Model file for the job. Use its own axes, mm. A direction names the side the tool comes from. Round coordinates to 2 decimals unless told otherwise and drop trailing zeros. Order: outer loops, then holes, each group sorted by start corner. A loop starts at its lowest first (then second) coordinate and runs counter-clockwise, first axis right, second up. Notation, with made-up numbers: (33, 57.25) -> (49, 57.25) arc R24 cw to (49, 70.25) -> close; hole circle Ø6 at (60, 89.5). An arc over 180 degrees is marked (long way). Put each result on its own line as item: value. Start each with the question number.
Q1. Cut at B-B, the plane x = 20. List the corners of the cut face in (y, z), and give its area (3 significant figures).
Q2. Cut at D-D, the plane x = 75. List the corners of the cut face in (y, z).
Q3. Pull direction Y, two halves, no side cores. Call faces 4 (the face through (31.45, -6.18, 6.44)), 5 (the face through (40.191, -13.594, 0.376)), 6 (the face through (62.31, -6.26, 7.31)): released by +Y, released by -Y, zero draft, split by the parting line, or undercut.
Q4. 3-axis set-ups, long thin cutter, end or side, ignore diameter. For faces 1 (the face through (13, 0, 6)), 2 (the face through (76, -6, 12.7)), 3 (the face through (69, 0, 6)): which of +Z, -Z, +X, -X, +Y, -Y reach the whole face in a straight line?
Q5. Probe L1, parallel to Z at x = 75, y = -6.5; L2, parallel to X at y = -6, z = 10.75; L3, parallel to X at y = -5, z = 6.35. List the from-to ranges inside material, lowest first.
Q6. Cut at A-A, the plane y = -6.35. State how many separate pieces and enclosed holes the cut face has, and give its area (3 significant figures).
Q7. Flat gauge pins, fed straight in: P1, Ø1, axis at x = 35, y = -11.5, coming from the +Z side; P2, Ø6.5, axis at x = 67.5, z = 7.5, coming from the +Y side; P3, Ø2, axis at y = -2.5, z = 3.5, coming from the -X side; P4, Ø4, axis at x = 60, z = 6.35, coming from the -Y side. Where does each tip first touch, or does it go through?
Q8. Cut at C-C, the plane x = 66. List the corners of the cut face in (y, z).
Autodesk Fusion 360 part; units mm, degrees
sketch "Screw Holes" plane through (0, 0, 0) normal (0, 1, 0) x (1, 0, 0)
  line L0 (0, 0) -> (80, 0)
  line L1 (80, 0) -> (80, -12.7)
  line L2 (80, -12.7) -> (0, -12.7)
  line L3 (0, -12.7) -> (0, 0)
  line L4 (0, -6.35) -> (80, -6.35) construction
  circle A0 centre (5, -6.35) radius 2
  circle A1 centre (20, -6.35) radius 2
  circle A2 centre (60, -6.35) radius 2.5
  circle A3 centre (75, -6.35) radius 2.5
  line L5 (5, -6.35) -> (0, -6.35)
  line L6 (75, -6.35) -> (80, -6.35)
  line L7 (5, -6.35) -> (20, -6.35) construction
  line L8 (60, -6.35) -> (75, -6.35) construction
  point P0 (67.5, -6.35)
  point P1 (12.5, -6.35)
  dimension "d1" = 80
  dimension "d2" = 12.7
  dimension "d3" = 4
  dimension "d4" = 4
  dimension "d5" = 5
  dimension "d6" = 5
  dimension "d7" = 40
  dimension "d8" = 15
  dimension "d9" = 15
extrude "Extrude1" add sketch "Screw Holes" against normal blind 12.7 contours A0 | A3 | L0 L1 L2 L3 | A1 | A2
extrude "Extrude2" cut sketch "Screw Holes" against normal through all contours A0 | A3 | A1 | A2
sketch "Loadcell Holes" plane through (0, 0, 12.7) normal (0, 0, 1) x (1, 0, 0)
  line L0 (80, 0) -> (0, 0)
  line L1 (0, 0) -> (0, -12.7)
  line L2 (0, -12.7) -> (80, -12.7)
  line L3 (80, -12.7) -> (80, 0)
  line L4 (40, -12.7) -> (40, 0) construction
  line L5 (0, -6.35) -> (80, -6.35) construction
  circle A0 centre (36.936, -6.35) radius 5.4886
  circle A1 centre (43.064, -6.35) radius 5.4886
  line L6 (36.936, -6.35) -> (43.064, -6.35)
extrude "Extrude3" cut sketch "Loadcell Holes" against normal blind 25 contours A0 A1 L6 | A0 A1 | A0 A1 L6 | A0 A1
sketch "Arrow" plane through (0, 0, 0) normal (-1, 0, 0) x (0, 0, 1)
  line L0 (12.7, 0) -> (0, 0)
  line L1 (0, 0) -> (0, -12.7)
  line L2 (0, -12.7) -> (12.7, -12.7)
  line L3 (12.7, -12.7) -> (12.7, 0)
  line L4 (5.511, -2.3504) -> (7.189, -2.3504)
  line L5 (7.189, -2.3504) -> (7.189, -8.0971)
  line L6 (7.189, -8.0971) -> (9.0409, -8.0971)
  line L7 (9.0409, -8.0971) -> (6.35, -10.7879)
  line L8 (6.35, -10.7879) -> (3.6591, -8.0971)
  line L9 (3.6591, -8.0971) -> (5.511, -8.0971)
  line L10 (5.511, -8.0971) -> (5.511, -2.3504)
  line L11 (6.35, -12.7) -> (6.35, 0) construction
  dimension "d20" = 45
extrude "Extrude4" cut sketch "Arrow" against normal blind 0.25 contours L4 L5 L6 L7 L8 L9 L10
sketch "Sketch5" plane through (0, 0, 0) normal (0, 1, 0) x (1, 0, 0)
  circle A0 centre (20, -6.35) radius 2
  circle A1 centre (60, -6.35) radius 2.5
  circle A2 centre (5, -6.35) radius 2
  circle A3 centre (75, -6.35) radius 2.5
  line L0 (80, -12.7) -> (80, 0)
  line L1 (80, 0) -> (0, 0)
  line L2 (0, 0) -> (0, -12.7)
  line L3 (0, -12.7) -> (80, -12.7)
  line L4 (40, 0) -> (40, -12.7) construction
  line L5 (26.35, 0) -> (53.65, 0)
  line L6 (53.65, 0) -> (53.65, -12.7)
  line L7 (53.65, -12.7) -> (26.35, -12.7)
  line L8 (26.35, -12.7) -> (26.35, 0)
  line L9 (26.35, -6.35) -> (40, -6.35) construction
  line L10 (40, -6.35) -> (53.65, -6.35) construction
  circle A4 centre (20, -6.35) radius 6.35 construction
extrude "Extrude6" add sketch "Sketch5" along normal blind 1.25 contours L1 L3 L5 L6 L7 L8
fillet "Fillet1" radius 1.25 4 edges at (26.35, 1.25, 6.35) (40, 1.25, 12.7) (53.65, 1.25, 6.35) (40, 1.25, 0)
sketch "Sketch6" plane through (0, -12.7, 0) normal (0, -1, 0) x (1, 0, 0)
  line L0 (80, 0) -> (80, 12.7)
  line L1 (80, 12.7) -> (0, 12.7)
  line L2 (0, 12.7) -> (0, 0)
  line L3 (0, 0) -> (80, 0)
  line L4 (26.35, 12.7) -> (26.35, 0)
  line L5 (26.35, 0) -> (0, 0)
  line L6 (0, 0) -> (0, 12.7)
  line L7 (0, 12.7) -> (26.35, 12.7)
  circle A0 centre (20, 6.35) radius 2
  circle A1 centre (5, 6.35) radius 2
  line L8 (53.65, 0) -> (53.65, 12.7)
  line L9 (53.65, 12.7) -> (80, 12.7)
  line L10 (80, 12.7) -> (80, 0)
  line L11 (80, 0) -> (53.65, 0)
  circle A2 centre (75, 6.35) radius 2.5
  circle A3 centre (60, 6.35) radius 2.5
  circle A4 centre (20, 6.35) radius 2
  circle A5 centre (60, 6.35) radius 2.5
  circle A6 centre (5, 6.35) radius 2
  circle A7 centre (75, 6.35) radius 2.5
  line L12 (5, 6.35) -> (20, 6.35) construction
  line L13 (60, 6.35) -> (75, 6.35) construction
  point P0 (67.5, 6.35)
  point P1 (12.5, 6.35)
extrude "Extrude7" add sketch "Sketch6" along normal blind 1.25 contours L1 L3 L4 L8
fillet "Fillet2" radius 1.25 4 edges at (26.35, -13.95, 6.35) (40, -13.95, 0) (53.65, -13.95, 6.35) (40, -13.95, 12.7)
sketch "Sketch7" plane through (0, 0, 12.7) normal (0, 0, 1) x (1, 0, 0)
  line L0 (26.35, -12.7) -> (53.65, -12.7)
  line L1 (53.65, -12.7) -> (80, -12.7)
  line L2 (80, -12.7) -> (80, 0)
  line L3 (80, 0) -> (53.65, 0)
  line L4 (53.65, 0) -> (26.35, 0)
  line L5 (26.35, 0) -> (0, 0)
  line L6 (0, 0) -> (0, -12.7)
  line L7 (0, -12.7) -> (26.35, -12.7)
  arc A0 (40, -1.7962) -> (40, -10.9038) centre (36.936, -6.35) ccw
  arc A1 (40, -10.9038) -> (40, -1.7962) centre (43.064, -6.35) ccw
  line L8 (51, 0) -> (72.1962, 0)
  line L9 (72.1962, 0) -> (72.1962, -12.7)
  line L10 (72.1962, -12.7) -> (51, -12.7)
  line L11 (51, -12.7) -> (51, 0)
extrude "Extrude8" add sketch "Sketch7" along normal blind 1.25 contours L0 L1 L3 L4 L8 L9 L10 L11
fillet "Fillet3" radius 1.25 4 edges at (51, -6.35, 13.95) (61.5981, 0, 13.95) (72.1962, -6.35, 13.95) (61.5981, -12.7, 13.95)
ref_plane "WorkPlane1" through (40, -6.975, 6.35) normal (0, 0, 1) x (-1, 0, 0)
ref_plane "WorkPlane2" through (65.5, -6.35, 6.975) normal (0, 1, 0) x (1, 0, 0)
ref_plane "WorkPlane3" through (40, -6.35, 6.35) normal (-1, 0, 0) x (0, 0, -1)
Ans:
1. outline: (-12.7, 0) -> (0, 0) -> (0, 4.35) -> (-12.7, 4.35) -> close; (-12.7, 8.35) -> (0, 8.35) -> (0, 12.7) -> (-12.7, 12.7) -> close
1. area: 110 mm^2
2. outline: (-12.7, 0) -> (0, 0) -> (0, 3.85) -> (-12.7, 3.85) -> close; (-12.7, 8.85) -> (0, 8.85) -> (0, 12.7) -> (-12.7, 12.7) -> close
3. face 4: undercut
3. face 5: released by -Y
3. face 6: zero draft
4. face 1: +Z, -Z, -X, +Y
4. face 2: +Z, +X, +Y, -Y
4. face 3: +Z, -Z, +X, +Y
5. L1: z = 0 to 3.85, 8.85 to 12.7
5. L2: x = 0 to 31.46, 48.54 to 80
5. L3: x = 0.25 to 3, 7 to 18, 22 to 31.62, 48.38 to 57.5, 62.5 to 72.5, 77.5 to 80
6. separate pieces: 2
6. enclosed holes: 4
6. area: 760 mm^2
7. P1: stops at z = 12.7
7. P2: stops at y = 0
7. P3: stops at x = 0
7. P4: passes through
8. outline: (-12.7, 0) -> (0, 0) -> (0, 12.7) arc R1.25 ccw to (-1.25, 13.95) -> (-11.45, 13.95) arc R1.25 ccw to (-12.7, 12.7) -> close
